Could you check a few things on this drawing? It's one solid part, dimensions in mm from its lowest x, y, z. A direction names the side the tool comes from. Round coordinates to 2 decimals unless told otherwise and drop trailing zeros. Loops run counter-clockwise (first coordinate to the right, second up) from the corner with the lowest first, then second, coordinate; pieces in that order, holes last. Notation, with made-up numbers: (-6.75, 1.5) -> (21.25, 1.5) arc R23 ccw to (21.25, 22.5) -> close; hole circle Ø7 at (-23, 35). An arc over 180 degrees is marked (long way). Write each question's results on one line, items separated by ' | '.
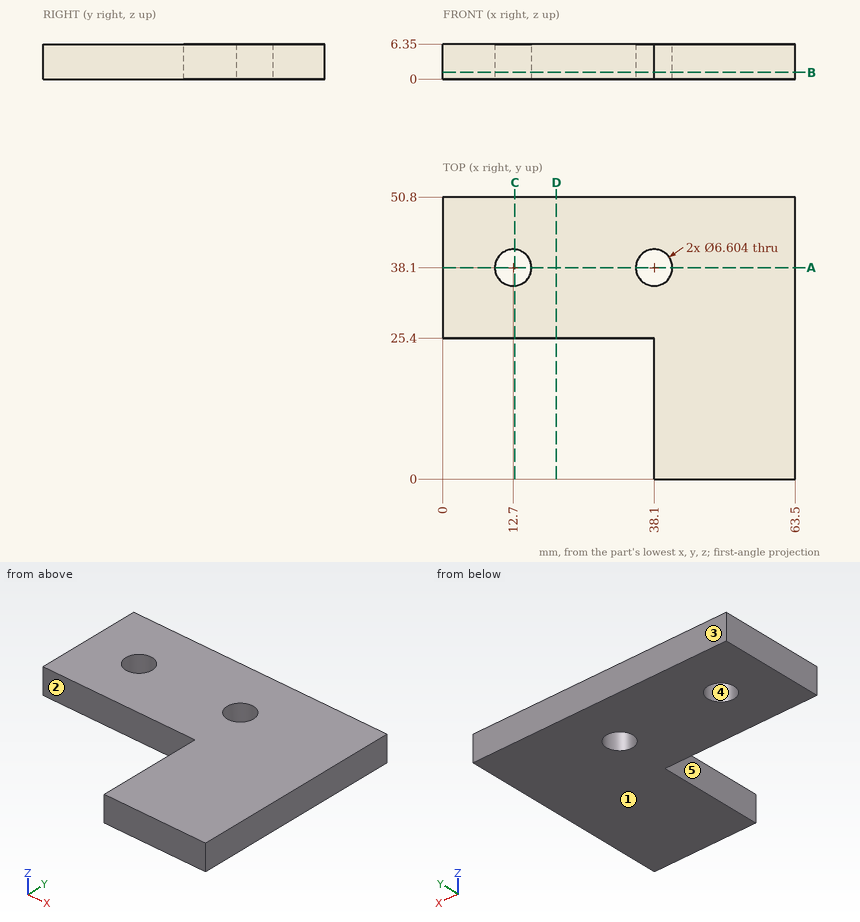
1) I want a section at B-B, the plane z = 1.25. Write out the boundary of the cut face in (x, y), plus the area to 3 significant figures.
Model answer:
outline: (0, 25.4) -> (38.1, 25.4) -> (38.1, 0) -> (63.5, 0) -> (63.5, 50.8) -> (0, 50.8) -> close; hole circle Ø6.6 at (12.7, 38.1); hole circle Ø6.6 at (38.1, 38.1) | area: 2,190 mm2
2) If we mould it in two halves opening along X, with no side actions, what happens to the marked faces 3, 4 and 5? For each: released by +X, released by -X, zero draft, split by the parting line, or undercut.
Model answer:
face 3: zero draft | face 4: undercut | face 5: released by -X
3) I want a section at D-D, the plane x = 20.5. Write out the boundary of the cut face in (y, z).
Model answer:
outline: (25.4, 0) -> (50.8, 0) -> (50.8, 6.35) -> (25.4, 6.35) -> close
4) I want a section at A-A, the plane y = 38.1. Write out the boundary of the cut face in (x, z), plus the area to 3 significant figures.
Model answer:
outline: (0, 0) -> (9.4, 0) -> (9.4, 6.35) -> (0, 6.35) -> close; (16, 0) -> (34.8, 0) -> (34.8, 6.35) -> (16, 6.35) -> close; (41.4, 0) -> (63.5, 0) -> (63.5, 6.35) -> (41.4, 6.35) -> close | area: 319 mm2
5) I want a section at C-C, the plane x = 13. Write out the boundary of the cut face in (y, z), plus the area to 3 significant figures.
Model answer:
outline: (25.4, 0) -> (34.81, 0) -> (34.81, 6.35) -> (25.4, 6.35) -> close; (41.39, 0) -> (50.8, 0) -> (50.8, 6.35) -> (41.39, 6.35) -> close | area: 120 mm2
6) I need wall thicknesses on line 1 (Y direction, x = 30, z = 0.5); line 2 (X direction, y = 7.5, z = 4.25); line 3 (Y direction, x = 14, z = 2.5) (1 decimal). Which ranges of each line are inside material? Lowest first, please.
Model answer:
line 1: y = 25.4 to 50.8 | line 2: x = 38.1 to 63.5 | line 3: y = 25.4 to 35.1, 41.1 to 50.8
7) For the marked faces 1 and 2, which set-ups out of +Z, -Z, +X, -X, +Y, -Y let a thin tool reach every point of the face, with its end or its side?
Model answer:
face 1: -Z, +X, -X, +Y, -Y | face 2: +Z, -Z, -X, -Y
8) I'm going to push a flat-ended pin straight in: pin 1 (5.5 mm diameter, centred on x = 12.7, y = 38.1, fed in from +Z). Where does the tip first touch, or does it pass through?
Model answer:
pin 1: passes through
